Geometry check sheet. Reference: the model listing, model coordinates, mm. Give positions to 0.01 mm unless a question says otherwise; leave off trailing zeros. Write each loop counter-clockwise with the first axis right and the second up, starting at its lowest first coordinate (ties: lowest second). Pieces come first, ordered by that corner, then holes. Notation, with made-up numbers: M 28.25,-10 L 41.25,-10 A13 cw 41.25,11 Z; hole C -29,46 d11. An arc over 180 degrees is marked long. One line per item, written item: value. Start each with the question number.
1. Cross-section at B-B on x = 8. Record the cut outline in (y, z).
2. Scan lines: line 1 (X direction, y = 1.65, z = 4.25); line 2 (Y direction, x = 11.5, z = 4.75); line 3 (X direction, y = 1.8, z = -9). Record each from-to range of solid material in increasing order.
3. Gauge pin test, flat ends, axial feed: pin 1 (1 mm diameter, centred on x = 11, z = -2, fed in from +Y); pin 2 (0.6 mm diameter, centred on x = 12.5, y = 1.5, fed in from -Z). Record the tip position at first contact, or that the pin passes through.
4. Cross-section at A-A on z = -4.25. Record the cut outline in (x, y).
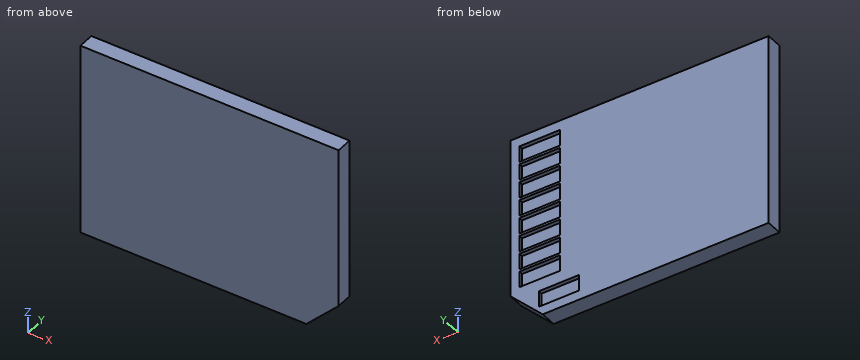
from build123d import *

# Parameters (mm, degrees)
SKETCH_1_W          = 32
SKETCH_1_H          = 24
EXTRUDE_1_DEPTH     = 2
CUT_EXTRUDE_1_DEPTH = 2
SKETCH_3_W          = 5
SKETCH_3_H          = 2
CUT_EXTRUDE_2_DEPTH = 0.5


with BuildPart() as part:
    # 草图1 → 拉伸1 (new body)
    with BuildSketch(Plane(origin=(0, 0, 0), x_dir=(1, 0, 0), z_dir=(0, 1, 0))):
        Rectangle(SKETCH_1_W, SKETCH_1_H)
    extrude(amount=EXTRUDE_1_DEPTH)

    # 草图2 → 切除-拉伸1 (cut)
    with BuildSketch(Plane(origin=(0, 2, 0), x_dir=(-1, 0, 0), z_dir=(0, 1, 0))):
        Polygon((-16, -12), (-12, -12), (-16, -8), align=None)
    extrude(amount=-CUT_EXTRUDE_1_DEPTH, mode=Mode.SUBTRACT)

    # 草图3 → 切除-拉伸2 (cut)
    with BuildSketch(Plane(origin=(0, 2, 0), x_dir=(-1, 0, 0), z_dir=(0, 1, 0))):
        with Locations((-12.385426295, 7.498304406)):
            Rectangle(SKETCH_3_W, SKETCH_3_H)
        with Locations((-12.385426295, 9.798304406)):
            Rectangle(SKETCH_3_W, SKETCH_3_H)
        with Locations((-12.385426295, 5.198304406)):
            Rectangle(SKETCH_3_W, SKETCH_3_H)
        with Locations((-12.385426295, 2.898304406)):
            Rectangle(SKETCH_3_W, SKETCH_3_H)
        with Locations((-12.385426295, 0.598304406)):
            Rectangle(SKETCH_3_W, SKETCH_3_H)
        with Locations((-12.385426295, -1.701695594)):
            Rectangle(SKETCH_3_W, SKETCH_3_H)
        with Locations((-12.385426295, -4.001695594)):
            Rectangle(SKETCH_3_W, SKETCH_3_H)
        with Locations((-12.385426295, -6.301695594)):
            Rectangle(SKETCH_3_W, SKETCH_3_H)
        with Locations((-9.977401753, -9.827028282)):
            Rectangle(SKETCH_3_W, SKETCH_3_H)
    extrude(amount=-CUT_EXTRUDE_2_DEPTH, mode=Mode.SUBTRACT)


solid = part.part
Report:
1. outline: M 0,-12 L 2,-12 L 2,-10.83 L 1.5,-10.83 L 1.5,-8.83 L 2,-8.83 L 2,12 L 0,12 Z
2. line 1: x = -16 to 9.89, 14.89 to 16
2. line 2: y = 0 to 1.5
2. line 3: x = -16 to 7.48, 12.48 to 15
3. pin 1: stops at y = 1.5
3. pin 2: stops at z = -11.8
4. outline: M -16,0 L 16,0 L 16,2 L 14.89,2 L 14.89,1.5 L 9.89,1.5 L 9.89,2 L -16,2 Z
